The model under review builds one solid part; all positions refer to its coordinate system, in mm. Coordinates: 2 decimals unless noted, no trailing zeros. Write each loop counter-clockwise with the first axis right and the second up, starting at its lowest first coordinate (ties: lowest second). Pieces come first, ordered by that corner, then holes. Notation, with made-up numbers: (80.25, 14.25) - (117.25, 14.25) arc R10 cw to (117.25, 25.25) - close; hole circle Ø11 at (79, 61.25). An arc over 180 degrees is marked (long way). Put each result on its own line as item: value. Start each with the question number.
Item 1: Consider section A-A on x = 0.2. Give the boundary of the cut face in (y, z).
Item 2: Consider section C-C on y = 18. Give the boundary of the cut face in (x, z), then the cut area to 3 significant figures.
Item 3: To check wall thickness, follow L1, parallel to Z at x = 0.2, y = 3.5; L2, parallel to X at y = 10.25, z = -0.35; L3, parallel to Z at x = 0.55, y = 14.5. State the ranges of each line that lie inside material, in increasing order. Write a range as [from, to].
Item 4: Consider section B-B on z = -0.4. Give the boundary of the cut face in (x, y), then the cut area to 3 significant figures.
Item 5: Consider section D-D on z = 0.35. Give the boundary of the cut face in (x, y).
```python
from build123d import *

# Parameters (mm, degrees)
TD_SKETCH_R                             = 0.79248
TL_FEATURE_DEPTH                        = 21.0312
TDF_STD_SKETCH_W                        = 2.09296
TDF_STD_SKETCH_H                        = 2.09296
TDF_STD_FEATURE_DEPTH                   = 22.061040395
ISA_20_STD_FEATURE_DEPTH                = 22.061040395
ISA_20_STD_FEATURE_DEPTH_BACK           = 22.061040395
F_10BA_STD_FEATURE_DEPTH                = 22.061040395
F_10BA_STD_FEATURE_DEPTH_BACK           = 22.061040395
FRO_STD_FEATURE_DEPTH                   = 22.061040395
FRO_STD_FEATURE_DEPTH_BACK              = 22.061040395
C_STD_FEATURE_DEPTH                     = 22.061040395
C_STD_FEATURE_DEPTH_BACK                = 22.061040395
ERW_STD_FEATURE_DEPTH                   = 0.01905
H_STD_FEATURE_REACH                     = 22.896
H_STD_SKETCH_R                          = 0.01905
H_STD_SKETCH_3_R                        = 0.01905
FUNNEL_FINAL_DIAMETRE_STD_FEATURE_DEPTH = 2.499995
FUNNEL_FINAL_DIAMETRE_STD_FEATURE_DRAFT = -13
ROUND_BR_STD_FEATURE_START              = -1
ROUND_BR_STD_FEATURE_DEPTH              = 1.009339363


with BuildPart() as part:
    # TD_sketch → TL_feature (new body)
    with BuildSketch(Plane(origin=(0, 0, 0), x_dir=(1, 0, 0), z_dir=(0, 1, 0))):
        with Locations(Location((0, 0, 0), (0, 0, 270))):
            Circle(TD_SKETCH_R)
    extrude(amount=TL_FEATURE_DEPTH)

    # TDF_STD_sketch → TDF_STD_feature (cut, through all)
    with BuildSketch(Plane(origin=(0, 0, 0), x_dir=(1, 0, 0), z_dir=(0, 1, 0))):
        with Locations((-1.4224, 0)):
            Rectangle(TDF_STD_SKETCH_W, TDF_STD_SKETCH_H)
    extrude(amount=TDF_STD_FEATURE_DEPTH, mode=Mode.SUBTRACT)

    # ISA_20_STD_sketch → ISA_20_STD_feature (cut, two sides: drawn at the far end of the back side and taken through both)
    with BuildSketch(Plane(origin=(0, 0, 0), x_dir=(0, 0, -1), z_dir=(1, 0, 0)).offset(-ISA_20_STD_FEATURE_DEPTH_BACK)):
        Polygon((-12.996080373, 73.27228267), (-3.784567997, 21.0312), (-0.0762, 0), (0.0762, 0), (3.784567997, 21.0312), (12.996080373, 73.27228267), (12.996080373, -32.821688483), (-12.996080373, -32.821688483), align=None)
    extrude(amount=ISA_20_STD_FEATURE_DEPTH + ISA_20_STD_FEATURE_DEPTH_BACK, mode=Mode.SUBTRACT)

    # 10BA_STD_sketch → 10BA_STD_feature (cut, two sides: drawn at the far end of the back side and taken through both)
    with BuildSketch(Plane.XY.offset(-F_10BA_STD_FEATURE_DEPTH_BACK)):
        Polygon((-53.216424634, 0), (-0.37592, 0), (-0.29972, 0), (-0.011354365, 0.050846642), (3.688047997, 21.0312), (12.863705333, 73.068938636), (91.245889802, 2.18375769), (25.165759835, -70.885180946), align=None)
    extrude(amount=F_10BA_STD_FEATURE_DEPTH + F_10BA_STD_FEATURE_DEPTH_BACK, mode=Mode.SUBTRACT)

    # FRO_STD_sketch → FRO_STD_feature (cut, two sides: drawn at the far end of the back side and taken through both)
    with BuildSketch(Plane.XY.offset(-FRO_STD_FEATURE_DEPTH_BACK)):
        with BuildLine():
            Line((-0.37592, 52.152138388), (-0.37592, 0.02794))
            ThreePointArc((-0.37592, 0.02794), (-0.367736563, 0.008183437), (-0.34798, 0))
            Line((-0.34798, 0), (51.776218388, 0))
            Line((51.776218388, 0), (-21.9385299, -73.714748288))
            Line((-21.9385299, -73.714748288), (-74.090668288, -21.5626099))
            Line((-74.090668288, -21.5626099), (-0.37592, 52.152138388))
        make_face()
    extrude(amount=FRO_STD_FEATURE_DEPTH + FRO_STD_FEATURE_DEPTH_BACK, mode=Mode.SUBTRACT)

    # C_STD_sketch → C_STD_feature (cut, two sides: drawn at the far end of the back side and taken through both)
    with BuildSketch(Plane(origin=(0, 0, 0), x_dir=(0, 0, -1), z_dir=(1, 0, 0)).offset(-C_STD_FEATURE_DEPTH_BACK)):
        with BuildLine():
            Line((-50.530423385, -12.791040855), (-0.030559272, 0))
            ThreePointArc((-0.030559272, 0), (0, 0.00381), (0.030559272, 0))
            Line((0.030559272, 0), (50.530423385, -12.791040855))
            Line((50.530423385, -12.791040855), (50.530423385, -116.980234183))
            Line((50.530423385, -116.980234183), (-50.530423385, -116.980234183))
            Line((-50.530423385, -116.980234183), (-50.530423385, -12.791040855))
        make_face()
    extrude(amount=C_STD_FEATURE_DEPTH + C_STD_FEATURE_DEPTH_BACK, mode=Mode.SUBTRACT)


with BuildPart() as body_2:
    # ERW_STD_sketch → ERW_STD_feature (new, symmetric)
    with BuildSketch(Plane.XY):
        Polygon((-0.1397, 0.09144), (-0.1397, 0), (-0.32512, 0), (-0.272327091, 0.09144), align=None)
    extrude(amount=ERW_STD_FEATURE_DEPTH, both=True)

    # H_STD_sketch → H_STD_feature (add, up to next)
    with BuildSketch(Plane(origin=(-0.010357492, 0.166115932, 0), x_dir=(0, 0, -1), z_dir=(0.8660254037844415, 0.4999999999999953, 0)), mode=Mode.PRIVATE) as h_std_feature_sk1:
        with Locations(Location((0, 0, 0), (0, 0, 90))):
            Circle(H_STD_SKETCH_R)
    h_std_feature_tool1 = extrude(h_std_feature_sk1.sketch, amount=-H_STD_FEATURE_REACH, mode=Mode.PRIVATE) - body_2.part
    add(h_std_feature_tool1.solids().sort_by_distance((-0.010357, 0.166116, 0))[0])


with BuildPart() as funnel_final_diametre_std_feature_tool:
    # H_STD_sketch<3> → funnel_final_diametre_STD_feature (with draft: the straight prism first)
    with BuildSketch(Plane(origin=(-0.010357492, 0.166115932, 0), x_dir=(0, 0, -1), z_dir=(0.8660254037844415, 0.4999999999999953, 0))):
        with Locations(Location((0, 0, 0), (0, 0, 90))):
            Circle(H_STD_SKETCH_3_R)
    extrude(amount=FUNNEL_FINAL_DIAMETRE_STD_FEATURE_DEPTH)
    # funnel_final_diametre_STD_feature: the draft: its side faces are tilted about the plane it starts from
    funnel_final_diametre_std_feature_sides = [funnel_final_diametre_std_feature_tool.faces().sort_by_distance(p)[0] for p in [
        (1.081697098, 0.774616898, 0),
    ]]
    draft(funnel_final_diametre_std_feature_sides, Plane(origin=(-0.010357492, 0.166115932, 0), x_dir=(0, 0, -1), z_dir=(0.8660254037844415, 0.4999999999999953, 0)), FUNNEL_FINAL_DIAMETRE_STD_FEATURE_DRAFT)


with BuildPart() as body_2_1:
    add(body_2.part)

    # funnel_final_diametre_STD_feature: add funnel_final_diametre_std_feature_tool
    add(funnel_final_diametre_std_feature_tool.part)

    # ROUND_BR_STD_feature: read off the stored shape, not the designer's step
    # ROUND_BR_STD_feature outline → ROUND_BR_STD_feature (cut)
    with BuildSketch(Plane(origin=(0, 0, 0), x_dir=(0.8660254037844362, -0.5000000000000042, 0), z_dir=(0.5000000000000042, 0.8660254037844363, 0)).offset(ROUND_BR_STD_FEATURE_START)):
        with BuildLine():
            Line((-0.281562179, -0.01905), (-0.262512179, -0.01905))
            ThreePointArc((-0.262512179, -0.01905), (-0.275982563, -0.013470384), (-0.281562179, 0))
            Line((-0.281562179, 0), (-0.281562179, -0.01905))
        make_face()
        with BuildLine():
            Line((-0.281562179, 0.01905), (-0.281562179, 0))
            ThreePointArc((-0.281562179, 0), (-0.275982563, 0.013470384), (-0.262512179, 0.01905))
            Line((-0.262512179, 0.01905), (-0.281562179, 0.01905))
        make_face()
    extrude(amount=ROUND_BR_STD_FEATURE_DEPTH, mode=Mode.SUBTRACT)


with BuildPart() as part_1:
    add(part.part)

    # COMBINE_STD_feature: cut body 2
    add(body_2_1.part, mode=Mode.SUBTRACT)


solid = part_1.part
```
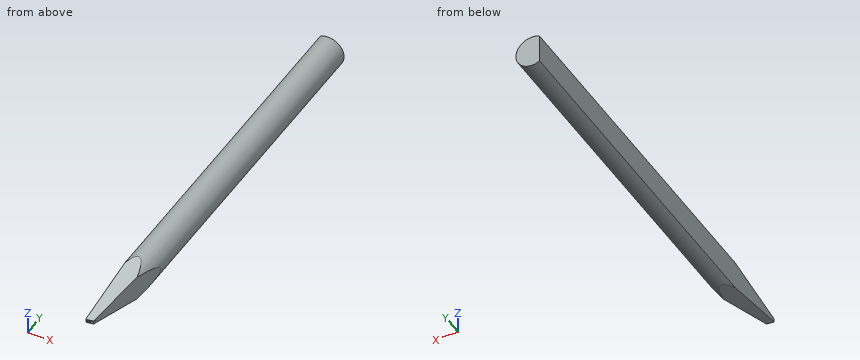
Report:
1. outline: (1.25, -0.3) - (3.92, -0.77) - (21.03, -0.77) - (21.03, 0.77) - (3.92, 0.77) - (1.25, 0.3) - close
2. outline: (-0.38, -0.7) arc R0.79 ccw (long way) to (-0.38, 0.7) - close
2. area: 1.56 mm²
3. L1: [-0.69, 0.69]
3. L2: [-0.38, 0.71]
3. L3: [-0.57, 0.57]
4. outline: (-0.38, 1.84) - (0.3, 1.84) - (0.68, 4) - (0.68, 21.03) - (-0.38, 21.03) - close
4. area: 19.9 mm²
5. outline: (-0.38, 1.55) - (0.25, 1.55) - (0.71, 4.15) - (0.71, 21.03) - (-0.38, 21.03) - close
